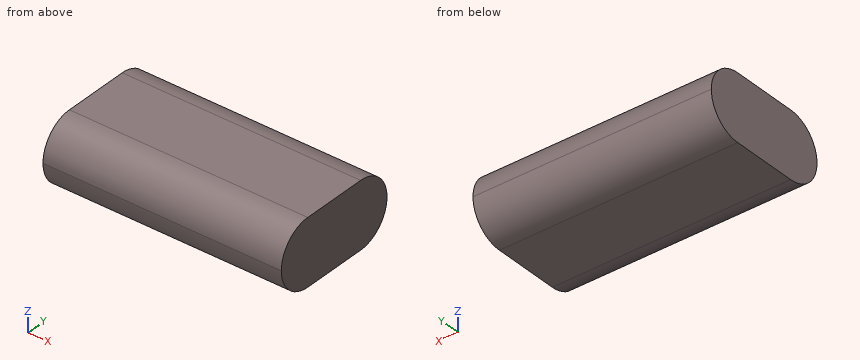
Autodesk Fusion 360 part; units mm, degrees
sketch "Sketch1" plane through (0, 0, 0) normal (0, 0, 1) x (1, 0, 0) in component "LiPo_Bat_4400_Dual_Cylinder"
  line L0 (33.5, 18.5) -> (-33.5, 18.5)
  line L1 (-33.5, 18.5) -> (-33.5, -18.5)
  line L2 (-33.5, -18.5) -> (33.5, -18.5)
  line L3 (33.5, -18.5) -> (33.5, 18.5)
  line L4 (33.5, 18.5) -> (-33.5, -18.5) construction
  line L5 (-33.5, 18.5) -> (33.5, -18.5) construction
  dimension "d1" = 67
  dimension "d2" = 37
extrude "Extrude1" add sketch "Sketch1" along normal blind 18.5 in component "LiPo_Bat_4400_Dual_Cylinder"
fillet "Fillet1" radius 9.25 4 edges at (0, -18.5, 18.5) (0, -18.5, 0) (0, 18.5, 0) (0, 18.5, 18.5) in component "LiPo_Bat_4400_Dual_Cylinder"
component "LiPo_Bat_4400_Dual_Cylinder" placed x (1, 0, 0) y (0, 1, 0) z (0, 0, 1) at (0, 0, 0)
Source: CAD feature listing. Evaluate the final solid. Frame: model axes, mm. Coordinates: 2 decimals unless noted, no trailing zeros. Loops run counter-clockwise (first coordinate to the right, second up) from the corner with the lowest first, then second, coordinate; pieces in that order, holes last. Notation, with made-up numbers: (54, 44) - (61, 44) arc R19 ccw to (61, 79) - close; hole circle Ø2 at (-11, 18.25). An arc over 180 degrees is marked (long way). One line per question, with ' | ' between items.
1) Section B-B, the plane z = 3.5. Return loops of the section in (x, y).
Report:
outline: (-33.5, -16.5) - (33.5, -16.5) - (33.5, 16.5) - (-33.5, 16.5) - close
2) First-contact query: P1, Ø1.5, axis at x = -17.5, z = 14, coming from the +Y side; P2, Ø3, axis at x = 26.5, z = 11, coming from the -Y side; P3, Ø1, axis at x = -18, y = -12.5, coming from the -Z side. Flat tips, straight axial feed; report the tip coordinate or a pass-through.
Report:
P1: stops at y = 17.59 | P2: stops at y = -18.5 | P3: stops at z = 0.42
3) Line query: line 1 along Y through (x, z) = (-23, 13.75); line 2 along Y through (x, z) = (3, 2); line 3 along Z through (x, y) = (3.5, -12). Output: solid intervals per line, ascending.
Report:
line 1: y = -17.33 to 17.33 | line 2: y = -15 to 15 | line 3: z = 0.42 to 18.08
4) Section C-C, the plane y = -13.5. Return loops of the section in (x, z), then the cut area to 3 significant figures.
Report:
outline: (-33.5, 1.03) - (33.5, 1.03) - (33.5, 17.47) - (-33.5, 17.47) - close | area: 1,100 mm²
